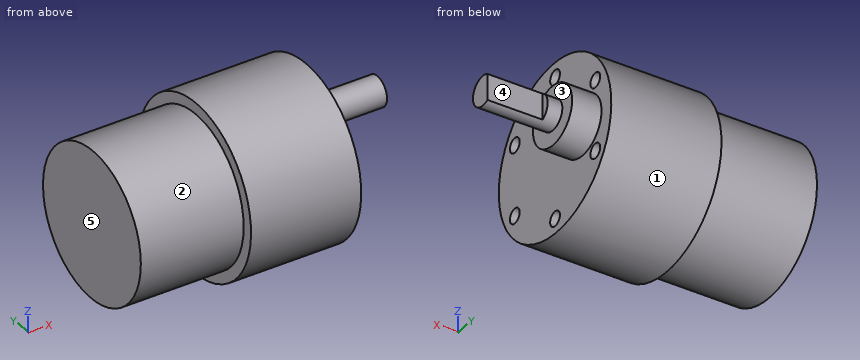
Autodesk Inventor part; units mm, degrees
ref_plane "YZ Plane" through (0, 0, 0) normal (1, 0, 0) x (0, 1, 0)
ref_plane "XZ Plane" through (0, 0, 0) normal (0, 1, 0) x (-1, 0, 0)
ref_plane "XY Plane" through (0, 0, 0) normal (0, 0, 1) x (1, 0, 0)
sketch "Sketch1" plane through (0, 0, 0) normal (1, 0, 0) x (0, 1, 0)
  circle A0 centre (0, 0) radius 15.875
  dimension "d0" = 31.75
extrude "Extrusion1" add sketch "Sketch1" along normal blind 22.225
sketch "Sketch2" plane through (22.225, 0, 0) normal (1, 0, 0) x (0, 0, -1)
  circle A0 centre (0, 0) radius 15.875 construction
  circle A1 centre (0, 0) radius 18.2563
  dimension "d3" = 36.5125
extrude "Extrusion2" add sketch "Sketch2" along normal blind 23.8125
sketch "Sketch3" plane through (46.0375, 0, 0) normal (1, 0, 0) x (0, 0, -1)
  circle A0 centre (0, 8.7313) radius 6.35
  circle A1 centre (0, 8.7313) radius 8.7313 construction
  line L0 (0, -25.5588) -> (0, 25.5588) construction
  point P0 (0, 0)
  dimension "d13" = 17.4625
  dimension "d7" = 12.7
extrude "Extrusion3" add sketch "Sketch3" along normal blind 6.35
sketch "Sketch4" plane through (52.3875, 8.7313, 0) normal (1, 0, 0) x (0, 0, -1)
  circle A0 centre (0, 0) radius 3.175
  circle A1 centre (0, 0) radius 6.35 construction
  point P0 (0, -8.7313)
  dimension "d10" = 6.35
extrude "Extrusion4" add sketch "Sketch4" along normal blind 15.0812
sketch "Sketch5" plane through (46.0375, 0, 0) normal (1, 0, 0) x (0, 0, -1)
  circle A0 centre (0, 0) radius 15.0812 construction
  line L0 (25.5588, 0) -> (-25.5588, 0) construction
  point P0 (15.0812, 0)
  dimension "d14" = 30.1625
hole "Hole1" at (46.0375, 0, -15.0812) direction (-1, 0, 0) diameter 3.175 depth 3.175
pattern_circular "Circular Pattern1" count 6 over 360 about axis through (-10, 0, 0) along (1, 0, 0) of "Hole1"
sketch "Sketch6" plane through (67.4687, 8.7313, 0) normal (1, 0, 0) x (0, 0, -1)
  circle A0 centre (0, 0) radius 3.175 construction
  line L0 (-2.7781, 1.5371) -> (2.7781, 1.5371)
  arc A1 (2.7781, 1.5371) -> (-2.7781, 1.5371) centre (0, 0) ccw
  point P0 (0, -8.7313)
  dimension "d25" = 5.5563
extrude "Extrusion5" cut sketch "Sketch6" against normal blind 11.9062
properties part number "Nextrox-Mini-12VDC-60rpmGearbox-Motor" material "Stainless Steel"
Geometry: final body of the model. Coordinates: model frame, mm. Face numbers are marked on the shaded views. A direction names the side the tool comes from. Round coordinates to 2 decimals unless told otherwise and drop trailing zeros. Loops run counter-clockwise (first coordinate to the right, second up) from the corner with the lowest first, then second, coordinate; pieces in that order, holes last. Notation, with made-up numbers: (85.25, 3.5) - (101.25, 3.5) arc R19 cw to (101.25, 20.5) - close; hole circle Ø9 at (44, -7.75). An arc over 180 degrees is marked (long way). Write each question's results on one line, items separated by ' | '. Start each with the question number.
1) Cut plane A-A on z = 0. Return loops of the section in (x, y) (1 decimal), then the cut area to 3 significant figures.
2) First-contact query: P1, Ø2.5, axis at y = 13, z = 7.5, coming from the +X side; P2, Ø1.5, axis at x = 38, y = -4.5, coming from the -Z side; P3, Ø8, axis at y = -1, z = 1, coming from the +X side. Flat tips, straight axial feed; report the tip coordinate or a pass-through.
3) Cut plane C-C on x = 6.5. Return loops of the section in (y, z) (3 decimals).
4) Cut plane B-B on y = -7.5. Return loops of the section in (x, z) (1 decimal), then the cut area to 3 significant figures.
5) Cut plane D-D on y = 0. Return loops of the section in (x, z) (1 decimal), then the cut area to 3 significant figures.
6) Access query for the marked faces 1, 2, 3, 4 and 5. Directions: +Z, -Z, +X, -X, +Y, -Y. A direction counts if a zero-diameter tool reaches every point of the face in a straight line with its end or side. Return the directions, or none.
7) Line query: probe 1 along X at (y, z) = (3.5, -3.5); probe 2 along X at (y, z) = (-15.5, 0.5); probe 3 along Z at (x, y) = (10, 0) (3 decimals). Output: solid intervals per line, ascending. Write a range as [from, to].
Verdict:
1) outline: (0, -15.9) - (22.2, -15.9) - (22.2, -18.3) - (46, -18.3) - (46, 2.4) - (52.4, 2.4) - (52.4, 5.6) - (67.5, 5.6) - (67.5, 10.3) - (55.6, 10.3) - (55.6, 11.9) - (52.4, 11.9) - (52.4, 15.1) - (46, 15.1) - (46, 18.3) - (22.2, 18.3) - (22.2, 15.9) - (0, 15.9) - close | area: 1,730 mm2
2) P1: stops at x = 42.86 | P2: stops at z = -17.87 | P3: stops at x = 52.39
3) outline: circle Ø31.75 at (0, 0)
4) outline: (0, -14) - (22.2, -14) - (22.2, -16.6) - (46, -16.6) - (46, 16.6) - (22.2, 16.6) - (22.2, 14) - (0, 14) - close | area: 1,410 mm2
5) outline: (0, -15.9) - (22.2, -15.9) - (22.2, -18.3) - (46, -18.3) - (46, -16.7) - (42.9, -16.7) - (42.9, -13.5) - (46, -13.5) - (46, 13.5) - (42.9, 13.5) - (42.9, 16.7) - (46, 16.7) - (46, 18.3) - (22.2, 18.3) - (22.2, 15.9) - (0, 15.9) - close | area: 1,550 mm2
6) face 1: +X, -X | face 2: -X | face 3: +X | face 4: +Z, -Z, +X, +Y | face 5: +Z, -Z, -X, +Y, -Y
7) probe 1: x = [0, 52.39] | probe 2: x = [0, 46.04] | probe 3: z = [-15.875, 15.875]
